Read the model definition and answer for the solid it produces. Units are mm, in the model's axes. A direction names the side the tool comes from. Give positions to 0.01 mm unless a question says otherwise; leave off trailing zeros. Order: outer loops, then holes, each group sorted by start corner. A loop starts at its lowest first (then second) coordinate and runs counter-clockwise, first axis right, second up. Notation, with made-up numbers: (70, 55.5) - (99, 55.5) arc R29 ccw to (99, 76.5) - close; hole circle Ø3 at (-7.5, -38). An arc over 180 degrees is marked (long way). Write each question's results on one line, items separated by ' | '. Start each with the question number.
Q1. A tool of negligible diameter and unlimited length cuts with its end or side. For faces 4 (the face through (1.11, 9.01, 16.01)), 5 (the face through (-8, -5, 5)), 6 (the face through (6.386, -0.575, 0.986)), 7 (the face through (6.386, -9.014, 4.425)), from which of +Z, -Z, +X, -X, +Y, -Y can it reach the whole face along a straight path? Write none if from no direction.
Q2. Flat-ended cylindrical pins translate along their axes: P1, Ø2.5, axis at y = 5, z = 5, coming from the -X side; P2, Ø1.5, axis at x = 0, z = 9.5, coming from the -Y side; P3, Ø1.5, axis at x = 5.5, y = 5.5, coming from the -Z side. Find the tip coordinate at first contact, or state that the pin passes through.
Q3. Find section B-B on x = 5. Give the vertices of the cut face in (y, z), and give its area (3 significant figures).
Q4. For a pull along X with two mould halves and no side action, classify faces 1 (the face through (9.038, 0.095, 0.913)), 2 (the face through (5.806, -3.735, 0.986)), 3 (the face through (0.095, 9.038, 0.913)) as +X half, -X half, draft (parallel to the pull), parting line (faces both ways), or undercut.
Q5. Find section D-D on y = 8.5. Give the vertices of the cut face in (x, z).
Q6. Find section A-A on y = 0. Give the vertices of the cut face in (x, z), and give its area (3 significant figures).
Q7. Find the intervals of material crossed by line 1 along Z through (x, y) = (-5, -9.55); line 2 along Y through (x, z) = (-8.25, 5.25); line 3 along Y through (x, z) = (-5, 1.4), in increasing order. Write a range as from..to.
from build123d import *

# Parameters (mm, degrees)
F0_W      = 20
F0_H      = 20
F1_DEPTH  = 20
F2_R      = 1.5
F3_DEPTH  = 2
F4_R      = 1.5
F5_DEPTH  = 2
F6_R      = 1.5
F7_DEPTH  = 2
F8_R      = 1.5
F9_DEPTH  = 2
F10_R     = 1.5
F11_DEPTH = 2
F12_R     = 1.5
F13_DEPTH = 2
F14_R     = 3.2


with BuildPart() as f1:
    # F0 (on Top) → F1 (new body)
    with BuildSketch(Plane.XY):
        Rectangle(F0_W, F0_H)
    extrude(amount=F1_DEPTH)

    # F2 (on face) → F3 (cut)
    with BuildSketch(Plane.XY):
        with Locations((-5, 5)):
            Circle(F2_R)
        with Locations((5, 5)):
            Circle(F2_R)
        with Locations((-5, 0)):
            Circle(F2_R)
        with Locations((5, 0)):
            Circle(F2_R)
        with Locations((-5, -5)):
            Circle(F2_R)
        with Locations((5, -5)):
            Circle(F2_R)
    extrude(amount=F3_DEPTH, mode=Mode.SUBTRACT)

    # F4 (on face) → F5 (cut)
    with BuildSketch(Plane.XY.offset(20)):
        Circle(F4_R)
    extrude(amount=-F5_DEPTH, mode=Mode.SUBTRACT)

    # F6 (on face) → F7 (cut)
    with BuildSketch(Plane.XZ.offset(10)):
        with Locations((0, 10)):
            Circle(F6_R)
        with Locations((-5, 5)):
            Circle(F6_R)
        with Locations((-5, 15)):
            Circle(F6_R)
        with Locations((5, 5)):
            Circle(F6_R)
        with Locations((5, 15)):
            Circle(F6_R)
    extrude(amount=-F7_DEPTH, mode=Mode.SUBTRACT)

    # F8 (on face) → F9 (cut)
    with BuildSketch(Plane(origin=(-10, 0, 0), x_dir=(0, -1, 0), z_dir=(-1, 0, 0))):
        with Locations((-5, 5)):
            Circle(F8_R)
        with Locations((-5, 15)):
            Circle(F8_R)
        with Locations((5, 5)):
            Circle(F8_R)
        with Locations((5, 15)):
            Circle(F8_R)
    extrude(amount=-F9_DEPTH, mode=Mode.SUBTRACT)

    # F10 (on face) → F11 (cut)
    with BuildSketch(Plane.YZ.offset(10)):
        with Locations((5, 5)):
            Circle(F10_R)
        with Locations((0, 10)):
            Circle(F10_R)
        with Locations((-5, 15)):
            Circle(F10_R)
    extrude(amount=-F11_DEPTH, mode=Mode.SUBTRACT)

    # F12 (on face) → F13 (cut)
    with BuildSketch(Plane(origin=(0, 10, 0), x_dir=(-1, 0, 0), z_dir=(0, 1, 0))):
        with Locations((0, 5)):
            Circle(F12_R)
        with Locations((0, 15)):
            Circle(F12_R)
    extrude(amount=-F13_DEPTH, mode=Mode.SUBTRACT)

    # F14
    f14_edges = [f1.edges().sort_by_distance(p)[0] for p in [
        (10, 0, 20),
        (10, 10, 10),
        (0, 10, 20),
        (10, -10, 10),
        (10, 0, 0),
        (0, 10, 0),
        (0, -10, 20),
        (-10, 0, 20),
        (0, -10, 0),
        (-10, 0, 0),
        (-10, -10, 10),
        (-10, 10, 10),
    ]]
    fillet(f14_edges, radius=F14_R)


solid = f1.part
Working result:
1) face 4: +Y | face 5: -X | face 6: -Z | face 7: -Y
2) P1: x = -8 | P2: y = -8 | P3: z = 2
3) outline: (-10, 3.2) arc R3.2 ccw to (-6.8, 0) - (-6.5, 0) - (-6.5, 2) - (-3.5, 2) - (-3.5, 0) - (-1.5, 0) - (-1.5, 2) - (1.5, 2) - (1.5, 0) - (3.5, 0) - (3.5, 2) - (6.5, 2) - (6.5, 0) - (6.8, 0) arc R3.2 ccw to (10, 3.2) - (10, 16.8) arc R3.2 ccw to (6.8, 20) - (-6.8, 20) arc R3.2 ccw to (-10, 16.8) - (-10, 16.5) - (-8, 16.5) - (-8, 13.5) - (-10, 13.5) - (-10, 6.5) - (-8, 6.5) - (-8, 3.5) - (-10, 3.5) - close | area: 361 mm²
4) face 1: +X half | face 2: undercut | face 3: draft
5) outline: (-9.51, 3.2) arc R2.71 ccw to (-6.8, 0.49) - (6.8, 0.49) arc R2.71 ccw to (9.51, 3.2) - (9.51, 16.8) arc R2.71 ccw to (6.8, 19.51) - (-6.8, 19.51) arc R2.71 ccw to (-9.51, 16.8) - close; hole circle Ø3 at (0, 5); hole circle Ø3 at (0, 15)
6) outline: (-10, 3.2) arc R3.2 ccw to (-6.8, 0) - (-6.5, 0) - (-6.5, 2) - (-3.5, 2) - (-3.5, 0) - (3.5, 0) - (3.5, 2) - (6.5, 2) - (6.5, 0) - (6.8, 0) arc R3.2 ccw to (10, 3.2) - (10, 8.5) - (8, 8.5) - (8, 11.5) - (10, 11.5) - (10, 16.8) arc R3.2 ccw to (6.8, 20) - (1.5, 20) - (1.5, 18) - (-1.5, 18) - (-1.5, 20) - (-6.8, 20) arc R3.2 ccw to (-10, 16.8) - close | area: 367 mm²
7) line 1: 1.56..3.5, 6.5..13.5, 16.5..18.44 | line 2: -9.65..-6.48, -3.52..3.52, 6.48..9.65 | line 3: -9.45..-6.5, -3.5..-1.5, 1.5..3.5, 6.5..9.45
